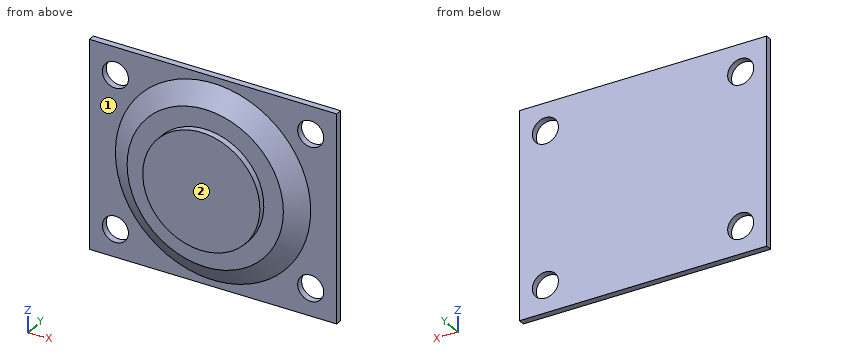
```python
from build123d import *

# Parameters (mm, degrees)
SKETCH1_W               = 38
SKETCH1_H               = 32
BOSS_EXTRUDE1_DEPTH     = 1
SKETCH2_R               = 2
CUT_EXTRUDE1_DEPTH      = 1
MIRROR2_COPY_1_SKETCH_R = 2
MIRROR2_COPY_1_DEPTH    = 1
SKETCH3_R               = 15
SKETCH4_R               = 12
SKETCH5_R               = 9
BOSS_EXTRUDE2_DEPTH     = 1


with BuildPart() as part:
    # Sketch1 → Boss-Extrude1 (new body)
    with BuildSketch(Plane(origin=(0, 0, 0), x_dir=(1, 0, 0), z_dir=(0, 1, 0))):
        Rectangle(SKETCH1_W, SKETCH1_H)
    extrude(amount=BOSS_EXTRUDE1_DEPTH)

    # Sketch2 → Cut-Extrude1 (cut)
    with BuildSketch(Plane(origin=(0, 1, 0), x_dir=(1, 0, 0), z_dir=(0, 1, 0))):
        with Locations(Location((15, -11.75, 0), (0, 0, 270))):
            Circle(SKETCH2_R)
    cut_extrude1 = extrude(amount=-CUT_EXTRUDE1_DEPTH, mode=Mode.SUBTRACT)

    # Mirror1: Cut-Extrude1 across plane
    add(cut_extrude1.mirror(Plane(origin=(0, 0, 0), x_dir=(0, 0, 1), z_dir=(1, 0, 0))), mode=Mode.SUBTRACT)

    # Mirror2: Cut-Extrude1 across plane
    add(cut_extrude1.mirror(Plane.XY), mode=Mode.SUBTRACT)

    # Mirror2 copy 1 sketch → Mirror2 copy 1 (cut)
    with BuildSketch(Plane(origin=(0, 1, 0), x_dir=(-1, 0, 0), z_dir=(0, 1, 0))):
        with Locations(Location((15, -11.75, 0), (0, 0, 270))):
            Circle(MIRROR2_COPY_1_SKETCH_R)
    extrude(amount=-MIRROR2_COPY_1_DEPTH, mode=Mode.SUBTRACT)

    # Sketch3 → Loft1 section 0
    with BuildSketch(Plane.XZ):
        Circle(SKETCH3_R)
    # Sketch4 → Loft1 section 1
    with BuildSketch(Plane.XZ.offset(2)):
        Circle(SKETCH4_R)
    loft()

    # Sketch5 → Boss-Extrude2 (add)
    with BuildSketch(Plane.XZ.offset(2)):
        with Locations(Location((0, 0, 0), (0, 0, 270))):
            Circle(SKETCH5_R)
    extrude(amount=BOSS_EXTRUDE2_DEPTH)


solid = part.part
```
Geometry: final body of the model. Coordinates: model frame, mm. Face numbers are marked on the shaded views. A direction names the side the tool comes from. Round coordinates to 2 decimals unless told otherwise and drop trailing zeros. Order: outer loops, then holes, each group sorted by start corner. A loop starts at its lowest first (then second) coordinate and runs counter-clockwise, first axis right, second up. Notation, with made-up numbers: M 16,50 L 43,50 A20 ccw 43,57 Z; hole C 85,-15 d11. An arc over 180 degrees is marked long. One line per item, written item: value.
(1) Cut plane B-B (x = 0). Return the cut outline in (y, z), and give its area (3 significant figures).
Result sheet:
outline: M -3,-9 L -2,-9 L -2,-12 L 0,-15 L 0,-16 L 1,-16 L 1,16 L 0,16 L 0,15 L -2,12 L -2,9 L -3,9 Z
area: 104 mm2
(2) Line query: probe 1 along X at (y, z) = (0.7, -11.75); probe 2 along Y at (x, z) = (16, 7); probe 3 along Y at (x, z) = (-8, 8.5). Output: solid intervals per line, ascending. Write a range as [from, to].
Result sheet:
probe 1: [-19, -17], [-13, 13], [17, 19]
probe 2: [0, 1]
probe 3: [-2, 1]
(3) Cut plane A-A (x = 15.5). Return the cut outline in (y, z).
Result sheet:
outline: M 0,-16 L 1,-16 L 1,-13.69 L 0,-13.69 Z; M 0,-9.81 L 1,-9.81 L 1,9.81 L 0,9.81 Z; M 0,13.69 L 1,13.69 L 1,16 L 0,16 Z
(4) Reachability of the marked faces 1 and 2 from +Z, -Z, +X, -X, +Y, -Y: full face, straight path, thin tool, end or side. Return the list, or none.
Result sheet:
face 1: -Y
face 2: +Z, -Z, +X, -X, -Y
(5) Cut plane C-C (z = 12.5). Give the number of separate pieces and of enclosed holes in the cut face, and give its area (3 significant figures).
Result sheet:
separate pieces: 3
enclosed holes: 0
area: 48.7 mm2
(6) Pin query (flat end, axial travel): P1, Ø1.5, axis at x = 7.5, y = -2.5, coming from the -Z side; P2, Ø1.5, axis at y = -1.5, z = 2.5, coming from the -X side; P3, Ø3, axis at x = -15, z = 11.75, coming from the +Y side; P4, Ø2, axis at x = 4.5, y = -2, coming from the +Z side. Return the tip coordinate at first contact, or that it passes through.
Result sheet:
P1: z = -9.95
P2: x = -13.66
P3: through
P4: z = 12.76
(7) Cut plane D-D (y = -1.5). Return the cut outline in (x, z), and give its area (3 significant figures).
Result sheet:
outline: C 0,0 d25.5
area: 511 mm2
